Design review of the part built by this model. Coordinates are the model's own, in mm. A direction names the side the tool comes from. Round coordinates to 2 decimals unless told otherwise and drop trailing zeros. Loops run counter-clockwise (first coordinate to the right, second up) from the corner with the lowest first, then second, coordinate; pieces in that order, holes last. Notation, with made-up numbers: (71.25, 43.25) - (91.25, 43.25) arc R17 cw to (91.25, 76.25) - close; hole circle Ø5 at (50.5, 36). An arc over 180 degrees is marked (long way). Return JSON: item names as keys, results as strings. Group by question number.
(1) The part is to be moulded in two halves that separate along Y. For faces 1 (the flat face through (-492, 0, -454)), 2 (the cylindrical face through (-423.95, -774.5, -346.87)), 3 (the flat face through (-424, -493, -577)), say which applies: pulls with the +Y half, pulls with the -Y half, needs draft (parallel to the pull), parting line crosses it, or undercut.
(2) Wall thickness on L1, parallel to Y at x = -425, z = -580; L2, parallel to X at y = -110, z = -453.5; L3, parallel to Z at x = -450, y = -190: over which ranges is each line inside the solid? List them lowest first. Write a range as [from, to].
(3) We need section A-A, the plane z = -462. Write out the cut boundary in (x, y).
(4) We need section B-B, the plane y = -80.5. Write out the cut boundary in (x, z).
(5) We need section C-C, the plane z = -378. Write out the cut boundary in (x, y).
(6) For faces 4 (the flat face through (-488, -493, -488)), 5 (the cylindrical face through (-493.986, -877.145, -344.703)), 6 (the cylindrical face through (-423.95, -225.877, -347.155)), 7 (the cylindrical face through (-436, -100, -583)), list the 3-axis set-ups (+Z, -Z, +X, -X, +Y, -Y) from which the entire face can be reached by the end or side of a thin tool; tool diameter is ignored.
(7) Clearance check with a flat-ended pin moving along its axis: pin 1 (17.5 mm diameter, centred on x = -425, y = -900, fed in from -Z). State where the tip first meets the part, or that it passes through.
(8) We need section D-D, the plane y = -718. Write out the cut boundary in (x, z), and give its area (3 significant figures).
from build123d import *

# Parameters (mm, degrees)
F1_DEPTH = 1000
F2_R     = 11
F3_DEPTH = 25
F5_DEPTH = 345


with BuildPart() as f1:
    # F0 (on Front) → F1 (new body)
    with BuildSketch(Plane.XZ):
        with BuildLine():
            ThreePointArc((-500, -568.999999), (-494.142136, -583.142134), (-480, -588.999999))
            Line((-480, -588.999999), (-370, -588.999999))
            ThreePointArc((-370, -588.999999), (-355.857864, -583.142134), (-350, -568.999999))
            Line((-350, -568.999999), (-350, -358.999999))
            ThreePointArc((-350, -358.999999), (-355.857864, -344.857863), (-370, -338.999999))
            Line((-370, -338.999999), (-480, -338.999999))
            ThreePointArc((-480, -338.999999), (-494.142136, -344.857863), (-500, -358.999999))
            Line((-500, -358.999999), (-500, -568.999999))
        make_face()
        with BuildLine():
            ThreePointArc((-488, -362.999999), (-484.485281, -354.514717), (-476, -350.999999))
            Line((-476, -350.999999), (-374, -350.999999))
            ThreePointArc((-374, -350.999999), (-365.514719, -354.514717), (-362, -362.999999))
            Line((-362, -362.999999), (-362, -564.999999))
            ThreePointArc((-362, -564.999999), (-365.514719, -573.48528), (-374, -576.999999))
            Line((-374, -576.999999), (-476, -576.999999))
            ThreePointArc((-476, -576.999999), (-484.485281, -573.48528), (-488, -564.999999))
            Line((-488, -564.999999), (-488, -362.999999))
        make_face(mode=Mode.SUBTRACT)
    extrude(amount=F1_DEPTH)

    # F2 (on face) → F3 (cut)
    with BuildSketch(Plane(origin=(0, 0, -588.999999), x_dir=(1, 0, 0), z_dir=(0, 0, -1))):
        with BuildLine():
            ThreePointArc((-425, 889), (-417.221825, 892.221825), (-414, 900))
            ThreePointArc((-414, 900), (-432.778175, 907.778175), (-425, 889))
        make_face()
        with Locations((-425, 100)):
            Circle(F2_R)
    extrude(amount=-F3_DEPTH, mode=Mode.SUBTRACT)

    # F4 (on face) → F5 (cut)
    with BuildSketch(Plane.YZ.offset(-350)):
        with BuildLine():
            ThreePointArc((-500, -438.999999), (-365.092624, -418.539985), (-242.318025, -358.999999))
            Line((-242.318025, -358.999999), (-500, -358.999999))
            Line((-500, -358.999999), (-500, -438.999999))
        make_face()
        with BuildLine():
            Line((-500, -358.999999), (-242.318025, -358.999999))
            ThreePointArc((-242.318025, -358.999999), (-228.672176, -349.24815), (-215.395011, -338.999999))
            Line((-215.395011, -338.999999), (-500, -338.999999))
            Line((-500, -338.999999), (-500, -358.999999))
        make_face()
        with BuildLine():
            Line((-500, -438.999999), (-500, -358.999999))
            Line((-500, -358.999999), (-757.681975, -358.999999))
            ThreePointArc((-757.681975, -358.999999), (-634.907376, -418.539985), (-500, -438.999999))
        make_face()
        with BuildLine():
            Line((-757.681975, -358.999999), (-500, -358.999999))
            Line((-500, -358.999999), (-500, -338.999999))
            Line((-500, -338.999999), (-784.604989, -338.999999))
            ThreePointArc((-784.604989, -338.999999), (-771.327824, -349.24815), (-757.681975, -358.999999))
        make_face()
        with BuildLine():
            Line((-500, -338.999999), (-215.395011, -338.999999))
            ThreePointArc((-215.395011, -338.999999), (-89.80476, -180.887949), (-45, 16.000001))
            ThreePointArc((-45, 16.000001), (-696.88795, 426.195241), (-784.604989, -338.999999))
            Line((-784.604989, -338.999999), (-500, -338.999999))
        make_face()
    extrude(amount=-F5_DEPTH, mode=Mode.SUBTRACT)


solid = f1.part
Solutions:
{
 "1": {"face 1": "pulls with the +Y half", "face 2": "undercut", "face 3": "needs draft"},
 "2": {"L1": "[-1000, -911], [-889, -111], [-89, 0]", "L2": "[-500, -488], [-362, -350]", "L3": "[-589, -577], [-351, -339]"},
 "3": {"outline": "(-500, -1000) - (-488, -1000) - (-488, 0) - (-500, 0) - close; (-362, -1000) - (-350, -1000) - (-350, 0) - (-362, 0) - close"},
 "4": {"outline": "(-500, -569) arc R20 ccw to (-480, -589) - (-370, -589) arc R20 ccw to (-350, -569) - (-350, -359) arc R20 ccw to (-370, -339) - (-480, -339) arc R20 ccw to (-500, -359) - close; hole (-488, -565) arc R12 ccw to (-476, -577) - (-374, -577) arc R12 ccw to (-362, -565) - (-362, -363) arc R12 ccw to (-374, -351) - (-476, -351) arc R12 ccw to (-488, -363) - close"},
 "5": {"outline": "(-500, -1000) - (-488, -1000) - (-488, -727.57) - (-500, -727.57) - close; (-500, -272.43) - (-488, -272.43) - (-488, 0) - (-500, 0) - close; (-362, -1000) - (-350, -1000) - (-350, -727.57) - (-362, -727.57) - close; (-362, -272.43) - (-350, -272.43) - (-350, 0) - (-362, 0) - close"},
 "6": {"face 4": "+Y, -Y", "face 5": "+Z, -X, +Y, -Y", "face 6": "+Z, +X, -X", "face 7": "-Z"},
 "7": {"pin 1": "z = -351"},
 "8": {"outline": "(-500, -569) arc R20 ccw to (-480, -589) - (-370, -589) arc R20 ccw to (-350, -569) - (-350, -383.38) - (-362, -383.38) - (-362, -565) arc R12 cw to (-374, -577) - (-476, -577) arc R12 cw to (-488, -565) - (-488, -383.38) - (-500, -383.38) - close", "area": "6,340 mm^2"}
}
